The drawing under review shows one solid part. Ordinate dimensions are in mm from its lowest x, y, z. A direction names the side the tool comes from. Coordinates: 2 decimals unless noted, no trailing zeros. Order: outer loops, then holes, each group sorted by start corner. A loop starts at its lowest first (then second) coordinate and runs counter-clockwise, first axis right, second up. Notation, with made-up numbers: M -27,-11.75 L -3,-11.75 A21 cw -3,27.25 Z; hole C 42,-15.75 d11. An arc over 180 degrees is marked long. Answer as a JSON object with one key per item and string values.
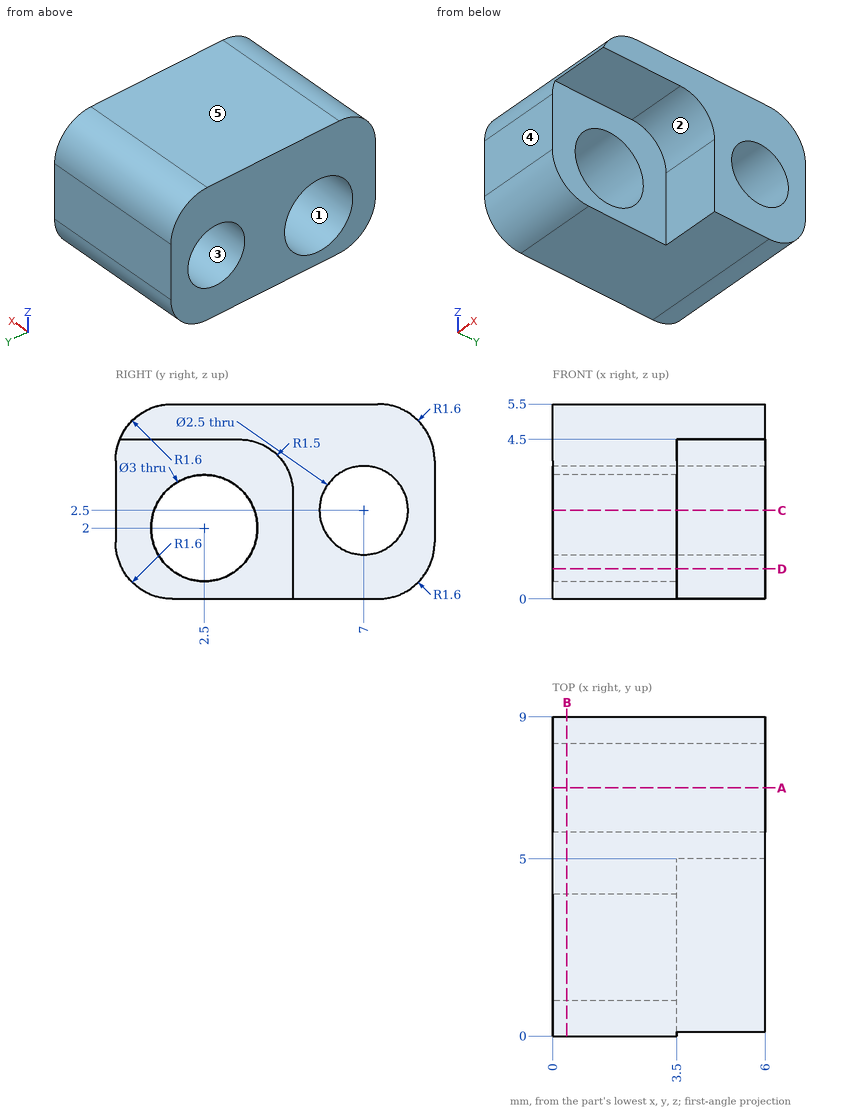
1) Add section B-B (x = 0.4). State the section outline as (y, z) points.
Taken from the geometry:
{"outline": "M 0,1.6 A1.6 ccw 1.6,0 L 7.4,0 A1.6 ccw 9,1.6 L 9,3.9 A1.6 ccw 7.4,5.5 L 1.6,5.5 A1.6 ccw 0,3.9 Z; hole C 2.5,2 d3; hole C 7,2.5 d2.5"}
2) Tool access review of the marked faces 1 and 2: name each direction out of +Z, -Z, +X, -X, +Y, -Y from which nothing blocks a thin tool from reaching the whole face with its end or side.
Taken from the geometry:
{"face 1": "+X, -X", "face 2": "-Z, +X, -Y"}
3) Insertion check: pin 1 Ø3 at (y, z) = (1, 1.5) entering from -X; pin 2 Ø2 at (x, y) = (5, 2) entering from -Z. Each pin has a flat end and moves straight along its axis. Give the tip position at first contact, or say it passes through.
Taken from the geometry:
{"pin 1": "stops at x = 0", "pin 2": "stops at z = 4.5"}
4) Add section C-C (z = 2.5). State the section outline as (x, y) points, and give its area (3 significant figures).
Taken from the geometry:
{"outline": "M 0,0 L 3.5,0 L 3.5,1.09 L 0,1.09 Z; M 0,3.91 L 3.5,3.91 L 3.5,5 L 6,5 L 6,5.75 L 0,5.75 Z; M 0,8.25 L 6,8.25 L 6,9 L 0,9 Z", "area": "16.6 mm2"}
5) To check wall thickness, follow L1, parallel to Y at x = 3.95, z = 2.5; L2, parallel to Z at x = 2.05, y = 2.5; L3, parallel to Y at x = 2.45, z = 2. State the ranges of each line that lie inside material, in increasing order.
Taken from the geometry:
{"L1": "y = 5 to 5.75, 8.25 to 9", "L2": "z = 0 to 0.5, 3.5 to 5.5", "L3": "y = 0 to 1, 4 to 5.85, 8.15 to 9"}
6) Add section A-A (y = 7). State the section outline as (x, z) points, and give its area (3 significant figures).
Taken from the geometry:
{"outline": "M 0,0 L 6,0 L 6,1.25 L 0,1.25 Z; M 0,3.75 L 6,3.75 L 6,5.5 L 0,5.5 Z", "area": "18.0 mm2"}
7) Add section D-D (z = 0.85). State the section outline as (x, y) points.
Taken from the geometry:
{"outline": "M 0,0.19 L 3.5,0.19 L 3.5,1.54 L 0,1.54 Z; M 0,3.46 L 3.5,3.46 L 3.5,5 L 6,5 L 6,8.81 L 0,8.81 Z"}
8) Mouldability with a two-part tool opening along Y and no side actions: class the marked faces 3, 4 and 5 as released by +Y, released by -Y, zero draft, split by the parting line, or undercut.
Taken from the geometry:
{"face 3": "undercut", "face 4": "released by -Y", "face 5": "zero draft"}
